Geometry: final body of the model. Coordinates: model frame, mm. A direction names the side the tool comes from. Coordinates: 2 decimals unless noted, no trailing zeros. Write each loop counter-clockwise with the first axis right and the second up, starting at its lowest first coordinate (ties: lowest second). Pieces come first, ordered by that corner, then holes. Notation, with made-up numbers: (61, -20.5) -> (94, -20.5) arc R18 cw to (94, 14.5) -> close; hole circle Ø4 at (-33.5, -18.75). An arc over 180 degrees is marked (long way). Answer as a JSON object with one key per item and string values. Group by question number.
```python
from build123d import *

# Parameters (mm, degrees)
SKETCH1_W           = 95.25
SKETCH1_H           = 69.85
BOSS_EXTRUDE1_DEPTH = 38.1
SKETCH2_W           = 88.9
SKETCH2_H           = 63.5
CUT_EXTRUDE1_DEPTH  = 31.75
CUT_EXTRUDE2_REACH  = 126.11
SKETCH3_W           = 6.35
SKETCH3_H           = 3.81
CUT_EXTRUDE3_REACH  = 126.11
SKETCH4_W           = 12.7
SKETCH4_H           = 5.08
SKETCH5_W           = 100.33
SKETCH5_H           = 74.93
BOSS_EXTRUDE2_DEPTH = 2.54


with BuildPart() as part:
    # Sketch1 → Boss-Extrude1 (new body)
    with BuildSketch(Plane(origin=(0, 0, 0), x_dir=(1, 0, 0), z_dir=(0, 1, 0))):
        with Locations((47.625, 34.925)):
            Rectangle(SKETCH1_W, SKETCH1_H)
    extrude(amount=BOSS_EXTRUDE1_DEPTH)

    # Sketch2 → Cut-Extrude1 (cut)
    with BuildSketch(Plane(origin=(0, 38.1, 0), x_dir=(1, 0, 0), z_dir=(0, 1, 0))):
        with Locations((47.625, 34.925)):
            Rectangle(SKETCH2_W, SKETCH2_H)
    extrude(amount=-CUT_EXTRUDE1_DEPTH, mode=Mode.SUBTRACT)

    # Sketch3 → Cut-Extrude2 (cut, up to next)
    with BuildSketch(Plane(origin=(95.25, 0, 0), x_dir=(0, 0, -1), z_dir=(1, 0, 0)), mode=Mode.PRIVATE) as cut_extrude2_sk1:
        with Locations((59.69, 10.795)):
            Rectangle(SKETCH3_W, SKETCH3_H)
    cut_extrude2_tool1 = extrude(cut_extrude2_sk1.sketch, amount=-CUT_EXTRUDE2_REACH, mode=Mode.PRIVATE) & part.part
    add(cut_extrude2_tool1.solids().sort_by_distance((95.25, 10.795, -59.69))[0], mode=Mode.SUBTRACT)

    # Sketch4 → Cut-Extrude3 (cut, up to next)
    with BuildSketch(Plane.ZY, mode=Mode.PRIVATE) as cut_extrude3_sk1:
        with Locations((-13.335, 24.13)):
            Rectangle(SKETCH4_W, SKETCH4_H)
    cut_extrude3_tool1 = extrude(cut_extrude3_sk1.sketch, amount=-CUT_EXTRUDE3_REACH, mode=Mode.PRIVATE) & part.part
    add(cut_extrude3_tool1.solids().sort_by_distance((0, 24.13, -13.335))[0], mode=Mode.SUBTRACT)

    # Sketch5 → Boss-Extrude2 (add)
    with BuildSketch(Plane.XZ):
        with Locations((47.625, -34.925)):
            Rectangle(SKETCH5_W, SKETCH5_H)
    extrude(amount=-BOSS_EXTRUDE2_DEPTH)


solid = part.part
```
Item 1: Section B-B on z = -35. Output: boundary loops of the cut face in (x, y) (3 decimals).
Item 2: Section C-C on y = 17. Output: boundary loops of the cut face in (x, z) (3 decimals).
Item 3: Section A-A on x = 75.5. Output: boundary loops of the cut face in (y, z) (3 decimals).
Item 4: Contact query for flat-ended pins moving along their axis: pin 1 (18 mm diameter, centred on x = 68.5, y = 20, fed in from +Z); pin 2 (1 mm diameter, centred on y = 19.5, z = -20, fed in from -X); pin 3 (19 mm diameter, centred on x = 45.5, z = -24.5, fed in from +Y). Output: stop coordinate, or through.
Item 5: Ray query, L1, parallel to X at y = 11, z = -21 (3 decimals); L2, parallel to Z at x = 27.5, y = 15 (3 decimals); L3, parallel to Y at x = 58.5, z = -14.5. Return the intervals inside material, ascending. Write a range as [from, to].
Item 6: Set-up query: faces 4 (the flat face through (47, 22, -66.675)), 5 (the flat face through (94, 8.89, -60)), 6 (the flat face through (47, 20, 0)), 7 (the flat face through (2, 21.59, -13)). Return all of +Z, -Z, +X, -X, +Y, -Y with unobstructed straight access to the full face (end or side cutting, diameter ignored); none if empty.
Item 7: Mould query, pull axis X, two halves, no side actions, for faces 1 (the flat face through (3.175, 22, -34)), 2 (the flat face through (2, 24, -19.685)), 3 (the flat face through (97.79, 1, -35)). Classes: +X half, -X half, draft (parallel to the pull), parting line (faces both ways), or undercut.
Answer sheet:
{
 "1": {"outline": "(-2.54, 0) -> (97.79, 0) -> (97.79, 2.54) -> (95.25, 2.54) -> (95.25, 38.1) -> (92.075, 38.1) -> (92.075, 6.35) -> (3.175, 6.35) -> (3.175, 38.1) -> (0, 38.1) -> (0, 2.54) -> (-2.54, 2.54) -> close"},
 "2": {"outline": "(0, -69.85) -> (95.25, -69.85) -> (95.25, 0) -> (0, 0) -> close; hole (3.175, -66.675) -> (92.075, -66.675) -> (92.075, -3.175) -> (3.175, -3.175) -> close"},
 "3": {"outline": "(0, -72.39) -> (2.54, -72.39) -> (2.54, -69.85) -> (38.1, -69.85) -> (38.1, -66.675) -> (6.35, -66.675) -> (6.35, -3.175) -> (38.1, -3.175) -> (38.1, 0) -> (2.54, 0) -> (2.54, 2.54) -> (0, 2.54) -> close"},
 "4": {"pin 1": "stops at z = 0", "pin 2": "stops at x = 0", "pin 3": "stops at y = 6.35"},
 "5": {"L1": "x = [0, 3.175], [92.075, 95.25]", "L2": "z = [-69.85, -66.675], [-3.175, 0]", "L3": "y = [0, 6.35]"},
 "6": {"face 4": "+Y", "face 5": "+X", "face 6": "+Z, +X, -X, +Y", "face 7": "-X"},
 "7": {"face 1": "undercut", "face 2": "draft", "face 3": "+X half"}
}
